from build123d import *

# Parameters (mm, degrees)
SKETCH1_R           = 2.65
BOSS_EXTRUDE1_DEPTH = 13
CUT_EXTRUDE1_DEPTH  = 48.895720059
FILLET1_R           = 2


with BuildPart() as part:
    # Sketch1 → Boss-Extrude1 (new body)
    with BuildSketch(Plane(origin=(0, 0, 0), x_dir=(1, 0, 0), z_dir=(0, 1, 0))):
        Polygon((-10, 10), (-10, -35), (10, -35), (10, -10), (30, -10), (30, 10), align=None)
        with Locations(Location((0, 0, 0), (0, 0, 90))):
            Circle(SKETCH1_R, mode=Mode.SUBTRACT)
        with Locations(Location((0, -27.5, 0), (0, 0, 90))):
            Circle(SKETCH1_R, mode=Mode.SUBTRACT)
        with Locations(Location((22.5, 0, 0), (0, 0, 90))):
            Circle(SKETCH1_R, mode=Mode.SUBTRACT)
    extrude(amount=BOSS_EXTRUDE1_DEPTH)

    # Sketch2 → Cut-Extrude1 (cut, through all)
    with BuildSketch(Plane(origin=(0, 13, 0), x_dir=(1, 0, 0), z_dir=(0, 1, 0))):
        Polygon((-7, -5.5), (4.792893219, -5.5), (7, -7.707106781), (7, -22), (-7, -22), align=None)
        Polygon((17, 7), (5.5, 7), (5.5, -4.792893219), (7.707106781, -7), (17, -7), align=None)
    extrude(amount=-CUT_EXTRUDE1_DEPTH, mode=Mode.SUBTRACT)

    # Fillet1
    fillet1_edges = [part.edges().sort_by_distance(p)[0] for p in [
        (30, 6.5, -10),
        (30, 6.5, 10),
        (10, 6.5, 10),
        (10, 6.5, 35),
        (-10, 6.5, 35),
        (-10, 6.5, -10),
        (7.707106781, 6.5, 7),
        (5.5, 6.5, 4.792893219),
        (5.5, 6.5, -7),
        (17, 6.5, -7),
        (17, 6.5, 7),
        (-7, 6.5, 22),
        (-7, 6.5, 5.5),
        (4.792893219, 6.5, 5.5),
        (7, 6.5, 7.707106781),
        (7, 6.5, 22),
    ]]
    fillet(fillet1_edges, radius=FILLET1_R)


solid = part.part
Read the model definition and answer for the solid it produces. Units are mm, in the model's axes. A direction names the side the tool comes from. Coordinates: 2 decimals unless noted, no trailing zeros. Write each loop counter-clockwise with the first axis right and the second up, starting at its lowest first coordinate (ties: lowest second). Pieces come first, ordered by that corner, then holes. Notation, with made-up numbers: (42, 51) -> (76, 51) arc R18 ccw to (76, 57) -> close; hole circle Ø2 at (-6.5, -25). An arc over 180 degrees is marked (long way). Return JSON: item names as keys, results as strings.
(1) The part is cut by section B-B on x = 22.5. Give the vertices of the cut face in (y, z).
Answers below:
{"outline": "(0, -10) -> (13, -10) -> (13, -2.65) -> (0, -2.65) -> close; (0, 2.65) -> (13, 2.65) -> (13, 10) -> (0, 10) -> close"}
(2) Each of these flat-tipped pins is pushed along its axis until it touches: P1, Ø10, axis at x = 5, z = 24.5, coming from the -Y side; P2, Ø6.5, axis at x = 17, y = 4, coming from the +Z side; P3, Ø5, axis at y = 10.5, z = 27.5, coming from the +X side; P4, Ø4, axis at x = 11, y = 7, coming from the +Z side. Where does it stop, or does it pass through?
Answers below:
{"P1": "y = 0", "P2": "z = 10", "P3": "x = 10", "P4": "z = 34.73"}
(3) For a pull along Z with two mould halves and no side action, classify faces 1 (the cylindrical face through (6.85, 6.41, 7.78)), 2 (the flat face through (-10, 6, 12)), 3 (the flat face through (20, 6, 10)) as pulls with the +Z half, pulls with the -Z half, needs draft (parallel to the pull), parting line crosses it, or undercut.
Answers below:
{"face 1": "undercut", "face 2": "needs draft", "face 3": "pulls with the +Z half"}
(4) The part is cut by section A-A on z = 27.5. Give the vertices of the cut face in (x, y).
Answers below:
{"outline": "(-10, 0) -> (-2.65, 0) -> (-2.65, 13) -> (-10, 13) -> close; (2.65, 0) -> (10, 0) -> (10, 13) -> (2.65, 13) -> close"}
(5) Consider line 1 along X through (y, z) = (9, 0); line 2 along Z through (x, y) = (3, 6.25); line 3 along Z through (x, y) = (22.5, 9.75). Determine where each line is inside the solid, lowest interval first. Write a range as from..to.
Answers below:
{"line 1": "-10..-2.65, 2.65..5.5, 17..19.85, 25.15..30", "line 2": "-10..5.5, 22..35", "line 3": "-10..-2.65, 2.65..10"}
(6) The part is cut by section D-D on x = -2. Give the vertices of the cut face in (y, z).
Answers below:
{"outline": "(0, -10) -> (13, -10) -> (13, -1.74) -> (0, -1.74) -> close; (0, 1.74) -> (13, 1.74) -> (13, 5.5) -> (0, 5.5) -> close; (0, 22) -> (13, 22) -> (13, 25.76) -> (0, 25.76) -> close; (0, 29.24) -> (13, 29.24) -> (13, 35) -> (0, 35) -> close"}
(7) Which of the six approach directions +Z, -Z, +X, -X, +Y, -Y give full straight-line access (tool end or side, diameter ignored) to faces 4 (the cylindrical face through (9.4, 6.59, 34.43)), 5 (the cylindrical face through (-6.43, 6.41, 21.4))?
Answers below:
{"face 4": "+Z, +X, +Y, -Y", "face 5": "+Y, -Y"}
(8) The part is cut by section C-C on z = 0. Give the vertices of the cut face in (x, y).
Answers below:
{"outline": "(-10, 0) -> (-2.65, 0) -> (-2.65, 13) -> (-10, 13) -> close; (2.65, 0) -> (5.5, 0) -> (5.5, 13) -> (2.65, 13) -> close; (17, 0) -> (19.85, 0) -> (19.85, 13) -> (17, 13) -> close; (25.15, 0) -> (30, 0) -> (30, 13) -> (25.15, 13) -> close"}
